Build history of the part. All positions in model axes, mm. A direction names the side the tool comes from. Give positions to 0.01 mm unless a question says otherwise; leave off trailing zeros. Loops run counter-clockwise (first coordinate to the right, second up) from the corner with the lowest first, then second, coordinate; pieces in that order, holes last. Notation, with made-up numbers: M 89.25,-14.5 L 110.25,-14.5 A13 cw 110.25,-6.5 Z; hole C 17.25,-14.75 d10. An arc over 180 degrees is marked long. Put each result on its own line as item: value.
```python
from build123d import *

# Parameters (mm, degrees)
SKETCH1_R               = 5
BOSS_EXTRUDE1_DEPTH     = 30
SKETCH3_R               = 10
BOSS_EXTRUDE3_DEPTH     = 10
SKETCH4_R               = 2
CUT_EXTRUDE1_DEPTH      = 11
CUT_EXTRUDE1_DEPTH_BACK = 11


with BuildPart() as part:
    # Sketch1 → Boss-Extrude1 (new body, symmetric)
    with BuildSketch(Plane.XY):
        Circle(SKETCH1_R)
    extrude(amount=BOSS_EXTRUDE1_DEPTH, both=True)

    # Sketch3 → Boss-Extrude3 (add)
    with BuildSketch(Plane.XY.offset(30)):
        Circle(SKETCH3_R)
    extrude(amount=BOSS_EXTRUDE3_DEPTH)

    # Sketch4 → Cut-Extrude1 (cut, two sides)
    with BuildSketch(Plane(origin=(0, 0, 0), x_dir=(0, 0, -1), z_dir=(1, 0, 0))) as cut_extrude1_sk:
        with Locations((-35, 0)):
            Circle(SKETCH4_R)
    extrude(amount=CUT_EXTRUDE1_DEPTH, mode=Mode.SUBTRACT)
    extrude(cut_extrude1_sk.sketch, amount=-CUT_EXTRUDE1_DEPTH_BACK, mode=Mode.SUBTRACT)


solid = part.part
```
Q1. Slice it at B-B (x = -8.5). List the corners of the cut face in (y, z).
Here are the results:
outline: M -5.27,30 L 5.27,30 L 5.27,40 L -5.27,40 Z; hole C 0,35 d4
Q2. Slice it at C-C (z = 35). List the corners of the cut face in (x, y), and give its area (3 significant figures).
Here are the results:
outline: M -9.8,-2 A10 ccw 9.8,-2 Z; M -9.8,2 L 9.8,2 A10 ccw Z
area: 235 mm²
Q3. Slice it at D-D (y = -2.75). List the corners of the cut face in (x, z).
Here are the results:
outline: M -9.61,30 L -4.18,30 L -4.18,-30 L 4.18,-30 L 4.18,30 L 9.61,30 L 9.61,40 L -9.61,40 Z
Q4. Probe line 1 (Z direction, x = 7, y = 0); line 2 (Z direction, x = 4.25, y = -7.5); line 3 (Y direction, x = -2, z = 35). List the from-to ranges inside material, lowest first. Write a range as from..to.
Here are the results:
line 1: 30..33, 37..40
line 2: 30..40
line 3: -9.8..-2, 2..9.8
Q5. Tool access for faces 1 (the flat face through (-5, -2, 30)), 2 (the flat face through (0, 0, -30)): list every direction of +Z, -Z, +X, -X, +Y, -Y with a clear straight run to the whole face (end or side of a thin tool).
Here are the results:
face 1: -Z
face 2: -Z, +X, -X, +Y, -Y
Q6. Slice it at A-A (y = 0). List the corners of the cut face in (x, z).
Here are the results:
outline: M -10,30 L -5,30 L -5,-30 L 5,-30 L 5,30 L 10,30 L 10,33 L -10,33 Z; M -10,37 L 10,37 L 10,40 L -10,40 Z
Q7. Drop flat-ended pins along their axis: pin 1 Ø8 at (x, z) = (-2.5, 8.5) entering from +Y; pin 2 Ø1 at (x, z) = (1, 17) entering from -Y. Give the stop position or say it passes through.
Here are the results:
pin 1: y = 5
pin 2: y = -4.97
Q8. Mould opens along Y. For faces 3 (the flat face through (0, 0, 40)), 4 (the cylindrical face through (-1.08, -4.88, 0.42)) say: pulls with the +Y half, pulls with the -Y half, needs draft (parallel to the pull), parting line crosses it, or undercut.
Here are the results:
face 3: needs draft
face 4: parting line crosses it
